Solid Edge part; units mm, degrees
sketch "Sketch1" plane through (0, 0, 0) normal (0, 0, 1) x (1, 0, 0)
  line L0 (447.68, 4.07) -> (19.9797, 4.07)
  arc A0 (17.0718, 3.1305) -> (19.9797, 4.07) centre (19.9797, -0.9) cw
  line L1 (4.359, -6.0417) -> (17.0718, 3.1305)
  arc A1 (0, 7.45) -> (4.359, -6.0417) centre (0, 0) ccw
  line L2 (0, 7.45) -> (253.3432, 7.45)
  arc A2 (253.3432, 7.45) -> (258.3132, 12.42) centre (253.3432, 12.42) ccw
  line L3 (258.3132, 408.38) -> (258.3132, 12.42)
  arc A3 (265.7632, 415.83) -> (258.3132, 408.38) centre (265.7632, 408.38) ccw
  line L4 (467.5797, 415.83) -> (265.7632, 415.83)
  arc A4 (467.5797, 415.83) -> (475.0297, 408.38) centre (467.5797, 408.38) cw
  line L5 (475.0297, 13.52) -> (475.0297, 408.38)
  arc A5 (475.0297, 13.52) -> (460.1514, 14.0875) centre (467.5797, 13.52) cw
  line L6 (460.1514, 14.0875) -> (462.8353, 49.2214)
  arc A6 (462.8353, 49.2214) -> (452.9183, 49.3079) centre (457.8797, 49.6) ccw
  line L7 (455.1171, 11.9578) -> (452.9183, 49.3079)
  arc A7 (447.68, 4.07) -> (455.1171, 11.9578) centre (447.68, 11.52) ccw
  line L8 (19.9797, 5.45) -> (447.68, 5.45)
  arc A8 (447.68, 5.45) -> (453.7395, 11.8767) centre (447.68, 11.52) ccw
  line L9 (451.5407, 49.2268) -> (453.7395, 11.8767)
  arc A9 (451.5407, 49.2268) -> (464.2113, 49.1163) centre (457.8797, 49.6) cw
  line L10 (464.2113, 49.1163) -> (461.5274, 13.9823)
  arc A10 (461.5274, 13.9823) -> (473.6497, 13.5199) centre (467.5797, 13.52) ccw
  line L11 (473.6573, 408.38) -> (473.6497, 13.5199)
  arc A11 (467.5797, 414.4576) -> (473.6573, 408.38) centre (467.5797, 408.38) cw
  line L12 (265.7632, 414.4576) -> (467.5797, 414.4576)
  arc A12 (259.6932, 408.38) -> (265.7632, 414.4576) centre (265.7708, 408.38) cw
  line L13 (259.6932, 12.42) -> (259.6932, 408.38)
  arc A13 (259.6932, 12.42) -> (253.3432, 6.07) centre (253.3432, 12.42) cw
  line L14 (253.3432, 6.07) -> (0, 6.07)
  arc A14 (3.5516, -4.9225) -> (0, 6.07) centre (0, 0) cw
  line L15 (16.2644, 4.2496) -> (3.5516, -4.9225)
  arc A15 (16.2644, 4.2496) -> (19.9797, 5.45) centre (19.9797, -0.9) cw
extrude "Protrusion1" add sketch "Sketch1" along normal blind 6
properties material "Polyurethene"
Here's how the part is built. I have some questions about the finished solid (model axes, mm). Give positions to 0.01 mm unless a question says otherwise; leave off trailing zeros. Loops run counter-clockwise (first coordinate to the right, second up) from the corner with the lowest first, then second, coordinate; pieces in that order, holes last. Notation, with made-up numbers: M 8.5,-24 L 23.5,-24 A23 cw 23.5,10 Z; hole C -7.75,67 d4. An arc over 180 degrees is marked long. Use one line per item in the form item = value. Start each with the question number.
Q1. If we section it at A-A (x = 293.5): Write out the boundary of the cut face in (y, z).
Q2. Will these pins go through, and if not, where does the flat tip stop? pin 1 Ø3 at (y, z) = (300, 3) entering from -X; pin 2 Ø3 at (x, z) = (81, 4.5) entering from -Y.
Q3. I need wall thicknesses on line 1 along X through (y, z) = (153, 2.3); line 2 along Y through (x, z) = (0, 1.2); line 3 along Y through (x, z) = (149, 4.5). Which ranges of each line are inside material? Lowest first, please.
Q4. If we section it at C-C (y = 328.5): Write out the boundary of the cut face in (x, z).
Q5. If we section it at D-D (y = 28.5): Write out the boundary of the cut face in (x, z).
Taken from the geometry:
q1.outline = M 4.07,0 L 5.45,0 L 5.45,6 L 4.07,6 Z; M 414.46,0 L 415.83,0 L 415.83,6 L 414.46,6 Z
q2.pin_1 = 258.31
q2.pin_2 = 4.07
q3.line_1 = 258.31 to 259.69, 473.65 to 475.03
q3.line_2 = -7.45 to -6.07, 6.07 to 7.45
q3.line_3 = 4.07 to 5.45, 6.07 to 7.45
q4.outline = M 258.31,0 L 259.69,0 L 259.69,6 L 258.31,6 Z; M 473.66,0 L 475.03,0 L 475.03,6 L 473.66,6 Z
q5.outline = M 258.31,0 L 259.69,0 L 259.69,6 L 258.31,6 Z; M 452.76,0 L 454.14,0 L 454.14,6 L 452.76,6 Z; M 461.25,0 L 462.64,0 L 462.64,6 L 461.25,6 Z; M 473.65,0 L 475.03,0 L 475.03,6 L 473.65,6 Z
